Could you check a few things on this model? Use its own coordinates, in mm. A direction names the side the tool comes from. Round coordinates to 2 decimals unless told otherwise and drop trailing zeros. Loops run counter-clockwise (first coordinate to the right, second up) from the corner with the lowest first, then second, coordinate; pieces in that order, holes last. Notation, with made-up numbers: (-26.5, -30) -> (4.5, -30) arc R26 cw to (4.5, 8) -> close; hole circle Ø11 at (54, 17). An arc over 180 degrees is marked (long way). One line per item, written item: value.
from build123d import *

# Parameters (mm, degrees)
SKETCH1_W                = 68.85
SKETCH1_H                = 107
BOSS_EXTRUDE1_DEPTH      = 2
SKETCH2_W                = 68.85
SKETCH2_H                = 2
BOSS_EXTRUDE2_DEPTH      = 67
CUT_EXTRUDE2_REACH       = 132.855
SKETCH5_W                = 68.85
SKETCH5_H                = 2
BOSS_EXTRUDE3_DEPTH      = 51
SKETCH6_W                = 68.85
SKETCH6_H                = 2
BOSS_EXTRUDE4_DEPTH      = 20.36
BOSS_EXTRUDE5_DEPTH      = 1.5
SKETCH13_W               = 2
SKETCH13_H               = 1.5
BOSS_EXTRUDE8_DEPTH      = 3
CUT_EXTRUDE4_REACH       = 97.75
SKETCH9_R                = 1.75
FILLET1_R                = 1.5
FILLET2_R                = 3
FILLET3_R                = 1.5
FILLET4_R                = 3
CUT_EXTRUDE5_REACH       = 111.975
SKETCH10_R               = 1.75
CHAMFER1_SIZE            = 2
SKETCH11_W               = 2
SKETCH11_H               = 109
BOSS_EXTRUDE6_DEPTH      = 4.5
SKETCH14_W               = 68.85
SKETCH14_H               = 0.5
BOSS_EXTRUDE9_DEPTH      = 2
FILLET5_R                = 2
FILLET6_R                = 4
FILLET8_R                = 4
CUT_EXTRUDE6_DEPTH       = 1
CUT_EXTRUDE7_DEPTH       = 125.986967721
SKETCH17_W               = 68.85
SKETCH17_H               = 2
BOSS_EXTRUDE10_DEPTH     = 8.66
SKETCH18_W               = 2
SKETCH18_H               = 68.16
BOSS_EXTRUDE11_DEPTH     = 2
SKETCH19_W               = 2
SKETCH19_H               = 68.16
BOSS_EXTRUDE12_DEPTH     = 2
FILLET9_R                = 4
FILLET10_R               = 4
FILLET11_R               = 1.5
BOSS_EXTRUDE13_START     = -2
BOSS_EXTRUDE13_OUTLINE_R = 1.6
BOSS_EXTRUDE13_DEPTH     = 2
BOSS_EXTRUDE14_START     = 19
SKETCH21_W               = 7.5
SKETCH21_H               = 1.5
BOSS_EXTRUDE14_DEPTH     = 4
CHAMFER2_SIZE            = 0.5
CHAMFER3_SIZE            = 0.75
SKETCH22_W               = 50
SKETCH22_H               = 2
CUT_EXTRUDE8_DEPTH       = 2
LPATTERN1_COUNT          = 4
LPATTERN1_PITCH          = 4.5


# Read off the part's stored shape, not the designer's step: Boss-Extrude13
with BuildPart() as part:
    # Sketch1 → Boss-Extrude1 (new body)
    with BuildSketch(Plane(origin=(0, 0, 0), x_dir=(1, 0, 0), z_dir=(0, 1, 0))):
        Rectangle(SKETCH1_W, SKETCH1_H)
    extrude(amount=BOSS_EXTRUDE1_DEPTH)

    # Sketch2 → Boss-Extrude2 (add)
    with BuildSketch(Plane.XZ):
        with Locations((0, -52.5)):
            Rectangle(SKETCH2_W, SKETCH2_H)
    extrude(amount=BOSS_EXTRUDE2_DEPTH)

    # Sketch4 → Cut-Extrude2 (cut, up to next)
    with BuildSketch(Plane(origin=(0, 0, -53.5), x_dir=(-1, 0, 0), z_dir=(0, 0, -1)), mode=Mode.PRIVATE) as cut_extrude2_sk1:
        Polygon((-2.25, -15.65), (-2.25, -20.95), (-0.15, -20.95), (-0.15, -15.65), (18.15, -15.65), (18.15, -35.75), (-20.55, -35.75), (-20.55, -15.65), align=None)
    cut_extrude2_tool1 = extrude(cut_extrude2_sk1.sketch, amount=-CUT_EXTRUDE2_REACH, mode=Mode.PRIVATE) & part.part
    add(cut_extrude2_tool1.solids().sort_by_distance((1.2, -25.807418, -53.5))[0], mode=Mode.SUBTRACT)

    # Sketch5 → Boss-Extrude3 (add)
    with BuildSketch(Plane.XY.offset(-51.5)):
        with Locations((0, -66)):
            Rectangle(SKETCH5_W, SKETCH5_H)
    extrude(amount=BOSS_EXTRUDE3_DEPTH)

    # Sketch6 → Boss-Extrude4 (add)
    with BuildSketch(Plane.XZ.offset(67)):
        with Locations((0, -1.5)):
            Rectangle(SKETCH6_W, SKETCH6_H)
    extrude(amount=BOSS_EXTRUDE4_DEPTH)

    # Sketch8 → Boss-Extrude5 (add)
    with BuildSketch(Plane(origin=(0, 2, 0), x_dir=(1, 0, 0), z_dir=(0, 1, 0))):
        Polygon((-36.425, 50.5), (-34.425, 50.5), (-34.425, -53.5), (34.425, -53.5), (34.425, 50.5), (36.425, 50.5), (36.425, -55.5), (-36.425, -55.5), align=None)
    extrude(amount=-BOSS_EXTRUDE5_DEPTH)

    # Sketch13 → Boss-Extrude8 (add)
    with BuildSketch(Plane(origin=(0, 0, -50.5), x_dir=(-1, 0, 0), z_dir=(0, 0, -1))):
        with Locations((35.425, 1.25)):
            Rectangle(SKETCH13_W, SKETCH13_H)
        with Locations((-35.425, 1.25)):
            Rectangle(SKETCH13_W, SKETCH13_H)
    extrude(amount=BOSS_EXTRUDE8_DEPTH)

    # Sketch9 → Cut-Extrude4 (cut, up to next)
    with BuildSketch(Plane.XZ.offset(67), mode=Mode.PRIVATE) as cut_extrude4_sk1:
        with Locations(Location((-25, -23.48, 0), (0, 0, 270))):
            Circle(SKETCH9_R)
    cut_extrude4_tool1 = extrude(cut_extrude4_sk1.sketch, amount=-CUT_EXTRUDE4_REACH, mode=Mode.PRIVATE) & part.part
    # Sketch9 → Cut-Extrude4 (cut, up to next)
    with BuildSketch(Plane.XZ.offset(67), mode=Mode.PRIVATE) as cut_extrude4_sk2:
        with Locations(Location((25, -23.48, 0), (0, 0, 270))):
            Circle(SKETCH9_R)
    cut_extrude4_tool2 = extrude(cut_extrude4_sk2.sketch, amount=-CUT_EXTRUDE4_REACH, mode=Mode.PRIVATE) & part.part
    add(cut_extrude4_tool1.solids().sort_by_distance((-25, -67, -23.48))[0], mode=Mode.SUBTRACT)
    add(cut_extrude4_tool2.solids().sort_by_distance((25, -67, -23.48))[0], mode=Mode.SUBTRACT)

    # Fillet1
    fillet1_edges = [part.edges().sort_by_distance(p)[0] for p in [
        (0, -67, -2.5),
    ]]
    fillet(fillet1_edges, radius=FILLET1_R)

    # Fillet2
    fillet2_edges = [part.edges().sort_by_distance(p)[0] for p in [
        (0, -65, -0.5),
    ]]
    fillet(fillet2_edges, radius=FILLET2_R)

    # Fillet3
    fillet3_edges = [part.edges().sort_by_distance(p)[0] for p in [
        (0, -65, -51.5),
    ]]
    fillet(fillet3_edges, radius=FILLET3_R)

    # Fillet4
    fillet4_edges = [part.edges().sort_by_distance(p)[0] for p in [
        (0, -67, -53.5),
    ]]
    fillet(fillet4_edges, radius=FILLET4_R)

    # Sketch10 → Cut-Extrude5 (cut, up to next)
    with BuildSketch(Plane.XY.offset(-0.5), mode=Mode.PRIVATE) as cut_extrude5_sk1:
        with Locations((-24.425, -79.36)):
            Circle(SKETCH10_R)
    cut_extrude5_tool1 = extrude(cut_extrude5_sk1.sketch, amount=-CUT_EXTRUDE5_REACH, mode=Mode.PRIVATE) & part.part
    # Sketch10 → Cut-Extrude5 (cut, up to next)
    with BuildSketch(Plane.XY.offset(-0.5), mode=Mode.PRIVATE) as cut_extrude5_sk2:
        with Locations((24.425, -79.36)):
            Circle(SKETCH10_R)
    cut_extrude5_tool2 = extrude(cut_extrude5_sk2.sketch, amount=-CUT_EXTRUDE5_REACH, mode=Mode.PRIVATE) & part.part
    add(cut_extrude5_tool1.solids().sort_by_distance((-24.425, -79.36, -0.5))[0], mode=Mode.SUBTRACT)
    add(cut_extrude5_tool2.solids().sort_by_distance((24.425, -79.36, -0.5))[0], mode=Mode.SUBTRACT)

    # Chamfer1
    chamfer1_edges = [part.edges().sort_by_distance(p)[0] for p in [
        (-34.425, -87.36, -1.5),
        (34.425, -87.36, -1.5),
    ]]
    chamfer(chamfer1_edges, length=CHAMFER1_SIZE)

    # Sketch11 → Boss-Extrude6 (add)
    with BuildSketch(Plane.XZ.offset(-0.5)):
        with Locations((35.425, 1)):
            Rectangle(SKETCH11_W, SKETCH11_H)
        with Locations((-35.425, 1)):
            Rectangle(SKETCH11_W, SKETCH11_H)
    extrude(amount=BOSS_EXTRUDE6_DEPTH)

    # Sketch14 → Boss-Extrude9 (add)
    with BuildSketch(Plane.XY.offset(53.5)):
        with Locations((0, 0.25)):
            Rectangle(SKETCH14_W, SKETCH14_H)
    extrude(amount=BOSS_EXTRUDE9_DEPTH)

    # Fillet5
    fillet5_edges = [part.edges().sort_by_distance(p)[0] for p in [
        (0, 0, -51.5),
        (34.425, 0, 2),
        (-34.425, 0, 2),
    ]]
    fillet(fillet5_edges, radius=FILLET5_R)

    # Fillet6
    fillet6_edges = [part.edges().sort_by_distance(p)[0] for p in [
        (0, 2, -53.5),
    ]]
    fillet(fillet6_edges, radius=FILLET6_R)

    # Fillet8
    # the kernel refuses this fillet: 4 mm, written as the material it takes off along each edge
    with BuildSketch(Plane(origin=(-36.425, 2, 65.5), x_dir=(1, 0, 0), z_dir=(0, 0, -1))) as fillet8_piece_1:
        with BuildLine():
            CenterArc((FILLET8_R, FILLET8_R), FILLET8_R, 180, 90)
            Line((0, FILLET8_R), (0, 0))
            Line((0, 0), (FILLET8_R, 0))
        make_face()
    extrude(amount=125, mode=Mode.SUBTRACT)
    with BuildSketch(Plane(origin=(36.425, 2, -59.5), x_dir=(0, -1, 0), z_dir=(0, 0, 1))) as fillet8_piece_2:
        with BuildLine():
            CenterArc((FILLET8_R, -FILLET8_R), FILLET8_R, 90, 90)
            Line((0, -FILLET8_R), (0, 0))
            Line((0, 0), (FILLET8_R, 0))
        make_face()
    extrude(amount=125, mode=Mode.SUBTRACT)

    # Sketch15 → Cut-Extrude6 (cut)
    with BuildSketch(Plane.XY.offset(55.5)):
        with BuildLine():
            Line((-36.425, -2), (-36.425, -4))
            Line((-36.425, -4), (-34.425, -4))
            Line((-34.425, -4), (-34.425, -2))
            ThreePointArc((-34.425, -2), (-33.839213562, -0.585786438), (-32.425, 0))
            Line((-32.425, 0), (32.425, 0))
            ThreePointArc((32.425, 0), (33.839213562, -0.585786438), (34.425, -2))
            Line((34.425, -2), (34.425, -4))
            Line((34.425, -4), (36.425, -4))
            Line((36.425, -4), (36.425, -2))
            ThreePointArc((36.425, -2), (35.253427125, 0.828427125), (32.425, 2))
            Line((32.425, 2), (-32.425, 2))
            ThreePointArc((-32.425, 2), (-35.253427125, 0.828427125), (-36.425, -2))
        make_face()
    extrude(amount=-CUT_EXTRUDE6_DEPTH, mode=Mode.SUBTRACT)

    # Sketch16 → Cut-Extrude7 (cut, through all)
    with BuildSketch(Plane(origin=(34.425, 0, 0), x_dir=(0, 0, -1), z_dir=(1, 0, 0))):
        with BuildLine():
            Line((2.5, -87.36), (0.5, -87.36))
            Line((0.5, -87.36), (0.5, -68))
            ThreePointArc((0.5, -68), (1.378679656, -65.878679656), (3.5, -65))
            Line((3.5, -65), (50, -65))
            ThreePointArc((50, -65), (51.060660172, -64.560660172), (51.5, -63.5))
            Line((51.5, -63.5), (53.5, -63.5))
            Line((53.5, -63.5), (53.5, -64))
            ThreePointArc((53.5, -64), (52.621320344, -66.121320344), (50.5, -67))
            Line((50.5, -67), (4, -67))
            ThreePointArc((4, -67), (2.939339828, -67.439339828), (2.5, -68.5))
            Line((2.5, -68.5), (2.5, -87.36))
        make_face()
    extrude(amount=-CUT_EXTRUDE7_DEPTH, mode=Mode.SUBTRACT)

    # Sketch17 → Boss-Extrude10 (add)
    with BuildSketch(Plane.XZ.offset(63.5)):
        with Locations((0, -52.5)):
            Rectangle(SKETCH17_W, SKETCH17_H)
    extrude(amount=BOSS_EXTRUDE10_DEPTH)

    # Sketch18 → Boss-Extrude11 (add)
    with BuildSketch(Plane(origin=(34.425, 0, 0), x_dir=(0, 0, -1), z_dir=(1, 0, 0))):
        with Locations((52.5, -38.08)):
            Rectangle(SKETCH18_W, SKETCH18_H)
    extrude(amount=BOSS_EXTRUDE11_DEPTH)

    # Sketch19 → Boss-Extrude12 (add)
    with BuildSketch(Plane.ZY.offset(34.425)):
        with Locations((-52.5, -38.08)):
            Rectangle(SKETCH19_W, SKETCH19_H)
    extrude(amount=BOSS_EXTRUDE12_DEPTH)

    # Fillet9
    fillet9_edges = [part.edges().sort_by_distance(p)[0] for p in [
        (36.425, -72.16, -52.5),
        (-36.425, -72.16, -52.5),
    ]]
    fillet(fillet9_edges, radius=FILLET9_R)

    # Fillet10
    fillet10_edges = [part.edges().sort_by_distance(p)[0] for p in [
        (35.425, -4, -51.5),
        (-35.425, -4, -51.5),
    ]]
    fillet(fillet10_edges, radius=FILLET10_R)

    # Fillet11
    fillet11_edges = [part.edges().sort_by_distance(p)[0] for p in [
        (35.425, -4, 54.5),
        (-35.425, -4, 54.5),
    ]]
    fillet(fillet11_edges, radius=FILLET11_R)

    # Boss-Extrude13 outline → Boss-Extrude13 (cut)
    with BuildSketch(Plane(origin=(0, 0, -53.5), x_dir=(-1, 0, 0), z_dir=(0, 0, -1)).offset(BOSS_EXTRUDE13_START)):
        with Locations((22, -64.16)):
            Circle(BOSS_EXTRUDE13_OUTLINE_R)
        with Locations((-22, -64.16)):
            Circle(BOSS_EXTRUDE13_OUTLINE_R)
    extrude(amount=BOSS_EXTRUDE13_DEPTH, mode=Mode.SUBTRACT)

    # Sketch21 → Boss-Extrude14 (add, symmetric)
    with BuildSketch(Plane(origin=(0, 0, 0), x_dir=(0, 0, -1), z_dir=(1, 0, 0)).offset(BOSS_EXTRUDE14_START)):
        with Locations((-52.25, -0.75)):
            Rectangle(SKETCH21_W, SKETCH21_H)
    boss_extrude14 = extrude(amount=BOSS_EXTRUDE14_DEPTH, both=True)

    # Mirror1: Boss-Extrude14 across plane
    add(boss_extrude14.mirror(Plane(origin=(0, 0, 0), x_dir=(0, 0, 1), z_dir=(1, 0, 0))))

    # Chamfer2
    chamfer2_edges = [part.edges().sort_by_distance(p)[0] for p in [
        (19, 0, 56),
        (-19, 0, 56),
    ]]
    chamfer(chamfer2_edges, length=CHAMFER2_SIZE)

    # Chamfer3
    chamfer3_edges = [part.edges().sort_by_distance(p)[0] for p in [
        (19, -1.5, 56),
        (-19, -1.5, 56),
    ]]
    chamfer(chamfer3_edges, length=CHAMFER3_SIZE)

    # Sketch22 → Cut-Extrude8 (cut)
    with BuildSketch(Plane(origin=(0, 2, 0), x_dir=(1, 0, 0), z_dir=(0, 1, 0))):
        with Locations((0, -46.5)):
            Rectangle(SKETCH22_W, SKETCH22_H)
    cut_extrude8 = extrude(amount=-CUT_EXTRUDE8_DEPTH, mode=Mode.SUBTRACT)

    # LPattern1: Cut-Extrude8 ×4
    with Locations(*[(0, 0, -i * LPATTERN1_PITCH) for i in range(1, LPATTERN1_COUNT)]):
        add(cut_extrude8, mode=Mode.SUBTRACT)


solid = part.part
(1) If we section it at C-C, the plane z = 23: Please give me the cut outline in (x, y) (3 decimals).
Recorded:
outline: (-36.425, -4) -> (-34.425, -4) -> (-34.425, -2) arc R2 cw to (-32.425, 0) -> (32.425, 0) arc R2 cw to (34.425, -2) -> (34.425, -4) -> (36.425, -4) -> (36.425, -2) arc R4 ccw to (32.425, 2) -> (-32.425, 2) arc R4 ccw to (-36.425, -2) -> close
(2) If I drill on L1, parallel to X at y = -64.16, z = -52.2 (3 decimals); L2, parallel to Y at x = -32.5, z = -29; L3, parallel to Z at x = 13, y = -50.5, over which ranges is the centre line in solid material (lowest first)?
Recorded:
L1: -36.425 to -23.6, -20.4 to 20.4, 23.6 to 36.425
L2: 0 to 2
L3: -53.5 to -51.5
(3) If we section it at D-D, the plane x = 29: Please give me the cut outline in (y, z).
Recorded:
outline: (-72.16, -53.5) -> (-2, -53.5) arc R4 ccw to (2, -49.5) -> (2, 54.5) -> (0, 54.5) -> (0, -49.5) arc R2 cw to (-2, -51.5) -> (-72.16, -51.5) -> close
(4) For faces 4 (the face through (0.51, 0.859, -52.297)), 5 (the face through (34.425, -3, 1)), which set-ups out of +Z, -Z, +X, -X, +Y, -Y let a thin tool reach every point of the face, with its end or its side?
Recorded:
face 4: -Z, +X, -X, +Y
face 5: +Z, -Y
(5) I'm going to push flat-ended pins straight in: pin 1 Ø1.6 at (x, z) = (35.5, -8.5) entering from -Y; pin 2 Ø1.6 at (x, y) = (-7.5, 1) entering from -Z; pin 3 Ø1.9 at (x, y) = (-22, -64.16) entering from -Z; pin 4 Ø1.6 at (y, z) = (0.5, 38) entering from -X. Where does each tip first touch, or does it pass through?
Recorded:
pin 1: y = -4
pin 2: z = -52.84
pin 3: through
pin 4: x = -36.05
(6) If we section it at A-A, the plane x = 11.5: Please give me the cut outline in (y, z), then the cut area to 3 significant figures.
Recorded:
outline: (-72.16, -53.5) -> (-35.75, -53.5) -> (-35.75, -51.5) -> (-72.16, -51.5) -> close; (-15.65, -53.5) -> (-2, -53.5) arc R4 ccw to (2, -49.5) -> (2, 32) -> (0, 32) -> (0, -49.5) arc R2 cw to (-2, -51.5) -> (-15.65, -51.5) -> close; (0, 34) -> (2, 34) -> (2, 36.5) -> (0, 36.5) -> close; (0, 38.5) -> (2, 38.5) -> (2, 41) -> (0, 41) -> close; (0, 43) -> (2, 43) -> (2, 45.5) -> (0, 45.5) -> close; (0, 47.5) -> (2, 47.5) -> (2, 54.5) -> (0, 54.5) -> close
area: 302 mm²
(7) If we section it at B-B, the plane y = -64.16: Please give me the cut outline in (x, z) (3 decimals).
Recorded:
outline: (-36.425, -53.5) -> (-23.6, -53.5) -> (-23.6, -51.5) -> (-36.425, -51.5) -> close; (-20.4, -53.5) -> (20.4, -53.5) -> (20.4, -51.5) -> (-20.4, -51.5) -> close; (23.6, -53.5) -> (36.425, -53.5) -> (36.425, -51.5) -> (23.6, -51.5) -> close
(8) Thinking about a two-plate mould opening in X: for faces 1 (the face through (19, -1.5, 52)), 2 (the face through (-35.28, 0.8, 1.26)), 3 (the face through (1, -38, -53.5)), which applies, released by +X, released by -X, zero draft, split by the parting line, or undercut?
Recorded:
face 1: undercut
face 2: released by -X
face 3: zero draft
